Can you work these out from the model? Positions are in its coordinate system, mm. A direction names the side the tool comes from. Round coordinates to 2 decimals unless told otherwise and drop trailing zeros. Loops run counter-clockwise (first coordinate to the right, second up) from the corner with the lowest first, then second, coordinate; pieces in that order, holes last. Notation, with made-up numbers: (-12, 43) - (15, 43) arc R31 cw to (15, 74) - close; hole circle Ø6 at (20, -7). An arc over 180 degrees is marked (long way). Answer as CSV lines item,"result".
```python
from build123d import *

# Parameters (mm, degrees)
F1_DEPTH  = 15
F2_W      = 12
F2_H      = 56
F3_DEPTH  = 48
F5_DEPTH  = 25
F7_DEPTH  = 36
F8_R      = 18
F8_R_2    = 11
F9_DEPTH  = 25
F11_DEPTH = 25


with BuildPart() as f1:
    # F0 (on Top) → F1 (new body)
    with BuildSketch(Plane.XY):
        with BuildLine():
            Line((-10.2415060103, 26.5643188208), (-41.7415060103, 26.5643188208))
            Line((-41.7415060103, 26.5643188208), (-41.7415060103, -1.4356811792))
            Line((-41.7415060103, -1.4356811792), (-31.9915060103, -1.4356811792))
            ThreePointArc((-31.9915060103, -1.4356811792), (-25.9915060103, 4.5643188208), (-19.9915060103, -1.4356811792))
            Line((-19.9915060103, -1.4356811792), (-10.2415060103, -1.4356811792))
            Line((-10.2415060103, -1.4356811792), (-10.2415060103, 26.5643188208))
        make_face()
        Polygon((1.7584939897, 26.5643188208), (-10.2415060103, 26.5643188208), (-10.2415060103, -1.4356811792), (-10.2415060103, -29.4356811792), (-4.2415060103, -29.4356811792), (1.7584939897, -29.4356811792), (1.7584939897, -1.4356811792), align=None)
        with BuildLine():
            Line((-31.9915060103, -1.4356811792), (-41.7415060103, -1.4356811792))
            Line((-41.7415060103, -1.4356811792), (-41.7415060103, -29.4356811792))
            Line((-41.7415060103, -29.4356811792), (-10.2415060103, -29.4356811792))
            Line((-10.2415060103, -29.4356811792), (-10.2415060103, -1.4356811792))
            Line((-10.2415060103, -1.4356811792), (-19.9915060103, -1.4356811792))
            ThreePointArc((-19.9915060103, -1.4356811792), (-25.9915060103, -7.4356811792), (-31.9915060103, -1.4356811792))
        make_face()
        with BuildLine():
            Line((33.2584939897, 26.5643188208), (1.7584939897, 26.5643188208))
            Line((1.7584939897, 26.5643188208), (1.7584939897, -1.4356811792))
            Line((1.7584939897, -1.4356811792), (11.5084939897, -1.4356811792))
            ThreePointArc((11.5084939897, -1.4356811792), (17.5084939897, 4.5643188208), (23.5084939897, -1.4356811792))
            Line((23.5084939897, -1.4356811792), (33.2584939897, -1.4356811792))
            Line((33.2584939897, -1.4356811792), (33.2584939897, 26.5643188208))
        make_face()
        with BuildLine():
            Line((11.5084939897, -1.4356811792), (1.7584939897, -1.4356811792))
            Line((1.7584939897, -1.4356811792), (1.7584939897, -29.4356811792))
            Line((1.7584939897, -29.4356811792), (33.2584939897, -29.4356811792))
            Line((33.2584939897, -29.4356811792), (33.2584939897, -1.4356811792))
            Line((33.2584939897, -1.4356811792), (23.5084939897, -1.4356811792))
            ThreePointArc((23.5084939897, -1.4356811792), (17.5084939897, -7.4356811792), (11.5084939897, -1.4356811792))
        make_face()
    extrude(amount=F1_DEPTH)

    # F2 (on face) → F3 (join)
    with BuildSketch(Plane.XY.offset(15)):
        with Locations((-4.2415060103, -1.4356811792)):
            Rectangle(F2_W, F2_H)
    extrude(amount=F3_DEPTH)

    # F4 (on face) → F5 (cut)
    with BuildSketch(Plane.YZ.offset(1.7584939897)):
        Polygon((-29.4356811792, 15), (26.5643188208, 63), (-29.4356811792, 63), align=None)
    extrude(amount=-F5_DEPTH, mode=Mode.SUBTRACT)

    # F6 (on face) → F7 (join)
    with BuildSketch(Plane(origin=(0, 26.5643188208, 0), x_dir=(-1, 0, 0), z_dir=(0, 1, 0))):
        Polygon((-1.7584939897, 63), (-1.7584939897, 15), (-1.7584939897, 0), (10.2415060103, 15), (10.2415060103, 63), align=None)
    extrude(amount=F7_DEPTH)

    # F8 (on face) → F9 (join)
    with BuildSketch(Plane.XY.offset(63)):
        with Locations((-4.2415060103, 62.5643188208)):
            Circle(F8_R)
        with Locations((-4.2415060103, 62.5643188208)):
            Circle(F8_R_2, mode=Mode.SUBTRACT)
    extrude(amount=-F9_DEPTH)

    # F10 (on face) → F11 (cut)
    with BuildSketch(Plane.YZ.offset(1.7584939897)):
        Polygon((45.5937560724, 38), (26.5643188208, 0), (62.5643188208, 0), (62.5643188208, 63), (53.3447743635, 63), (53.3447743635, 38), align=None)
    extrude(amount=-F11_DEPTH, mode=Mode.SUBTRACT)


solid = f1.part
```
Q1. On a 3-axis mill with a long thin cutter (end or side, diameter ignored), from which of +Z, -Z, +X, -X, +Y, -Y can I reach the whole of each face in a straight line? I mean faces 1 (the flat face through (18, 26.564, 7)), 2 (the flat face through (-9, 53.345, 51)), 3 (the flat face through (-10.242, 16, 33)), 4 (the flat face through (-6.8, 28.6, 10.7)), 5 (the flat face through (-26, 5, 15)). Say none if no direction works.
Checks:
face 1,"+Z, -Z, +X, +Y"
face 2,"+Z, -Z, -X"
face 3,"+Z, -X, -Y"
face 4,"-Z, -X, +Y"
face 5,"+Z, -X, +Y, -Y"
Q2. We'd pull the mould along Y, two halves only. Please class faces 6 (the flat face through (4, 71, 38)), 7 (the cylindrical face through (-15.72, 48.7, 50.68)), 8 (the flat face through (-25, 26.564, 7)), 9 (the flat face through (-19, 62.564, 50)): pulls with the +Y half, pulls with the -Y half, needs draft (parallel to the pull), parting line crosses it, or undercut.
Checks:
face 6,"needs draft"
face 7,"pulls with the -Y half"
face 8,"pulls with the +Y half"
face 9,"undercut"
Q3. Imagine slicing it at A-A (x = -13). Write out the boundary of the cut face in (y, z), then the cut area to 3 significant figures.
Checks:
outline,"(-29.44, 0) - (26.56, 0) - (26.56, 15) - (-29.44, 15) - close; (46.84, 38) - (53.34, 38) - (53.34, 63) - (46.84, 63) - close; (69.22, 38) - (78.29, 38) - (78.29, 63) - (69.22, 63) - close"
area,"1,230 mm²"
Q4. I'm going to push flat-ended pins straight in: pin 1 Ø6 at (x, z) = (8, 37) entering from -Y; pin 2 Ø12 at (y, z) = (6.5, 23) entering from -X; pin 3 Ø16.5 at (x, z) = (22, 5) entering from +Y; pin 4 Ø6 at (x, y) = (5.5, 39) entering from +Z. Where does each tip first touch, or does it pass through?
Checks:
pin 1,"y = 47.22"
pin 2,"x = -10.24"
pin 3,"y = 26.56"
pin 4,"through"
Q5. Imagine slicing it at D-D (z = 54). Write out the boundary of the cut face in (x, y).
Checks:
outline,"(-22.24, 62.56) - (-15.24, 62.56) arc R11 cw (long way) to (1.76, 53.34) - (-19.7, 53.34) arc R18 ccw to (-10.24, 45.59) - (-10.24, 16.06) - (1.76, 16.06) - (1.76, 45.59) arc R18 ccw (long way) to start"
Q6. If I drill on line 1 along Z through (x, y) = (-20, 25); line 2 along X through (y, z) = (39.5, 51.5); line 3 along Y through (x, z) = (17.5, 10.5), over which ranges is the centre line in solid material (lowest first)? Write a range as [from, to].
Checks:
line 1,"[0, 15]"
line 2,"[-10.24, 1.76]"
line 3,"[-29.44, -7.44], [4.56, 26.56]"
Q7. Imagine slicing it at B-B (x = 16.5). Write out the boundary of the cut face in (y, z).
Checks:
outline,"(-29.44, 0) - (-7.35, 0) - (-7.35, 15) - (-29.44, 15) - close; (4.48, 0) - (26.56, 0) - (26.56, 15) - (4.48, 15) - close"
Q8. Imagine slicing it at C-C (y = 68). Write out the boundary of the cut face in (x, z), then the cut area to 3 significant figures.
Checks:
outline,"(-21.4, 38) - (-13.8, 38) - (-13.8, 63) - (-21.4, 63) - close; (5.32, 38) - (12.92, 38) - (12.92, 63) - (5.32, 63) - close"
area,"380 mm²"
